Can you work these out from the drawing? Everything is in mm from the part's minimum corner. A direction names the side the tool comes from. Give positions to 0.01 mm unless a question says otherwise; leave off trailing zeros. Order: outer loops, then holes, each group sorted by start corner. A loop starts at its lowest first (then second) coordinate and runs counter-clockwise, first axis right, second up. Notation, with made-up numbers: M -19.75,49.5 L 36.25,49.5 A22 ccw 36.25,81.5 Z; hole C 81,38.25 d8. An arc over 180 degrees is marked long. Answer as a JSON object with one key per item and string values.
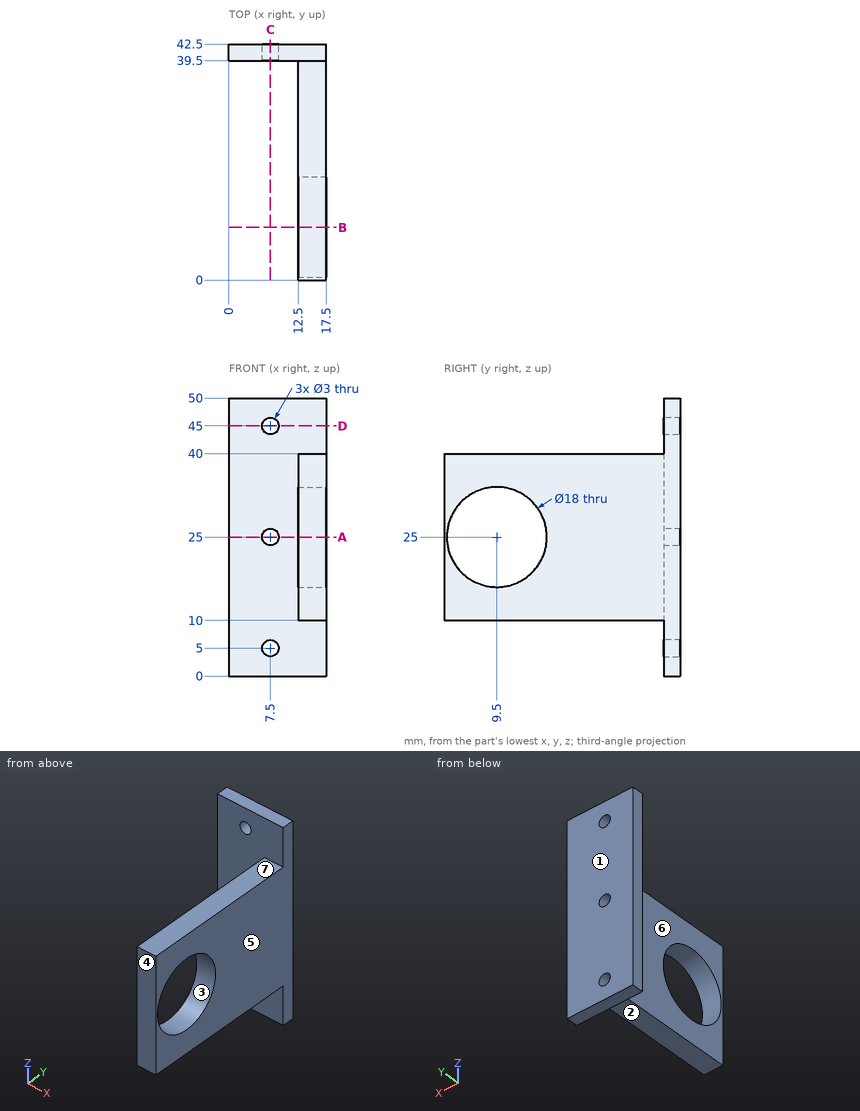
1) I want a section at A-A on z = 25. Write out the boundary of the cut face in (x, y).
Results found:
{"outline": "M 0,39.5 L 6,39.5 L 6,42.5 L 0,42.5 Z; M 9,39.5 L 12.5,39.5 L 12.5,18.5 L 17.5,18.5 L 17.5,42.5 L 9,42.5 Z; M 12.5,0 L 17.5,0 L 17.5,0.5 L 12.5,0.5 Z"}
2) For the marked faces 5, 6 and 7, which set-ups out of +Z, -Z, +X, -X, +Y, -Y let a thin tool reach every point of the face, with its end or its side?
Results found:
{"face 5": "+Z, -Z, +X, +Y, -Y", "face 6": "+Z, -Z, -X, -Y", "face 7": "+Z, +X, -X, -Y"}
3) I want a section at D-D on z = 45. Write out the boundary of the cut face in (x, y).
Results found:
{"outline": "M 0,39.5 L 6,39.5 L 6,42.5 L 0,42.5 Z; M 9,39.5 L 17.5,39.5 L 17.5,42.5 L 9,42.5 Z"}
4) I'm going to push flat-ended pins straight in: pin 1 Ø14.5 at (y, z) = (9.5, 25) entering from +X; pin 2 Ø1.5 at (x, y) = (16, 13) entering from -Z; pin 3 Ø2.5 at (x, y) = (14, 11.5) entering from +Z; pin 4 Ø24 at (y, z) = (10, 21.5) entering from -X. Where does each tip first touch, or does it pass through?
Results found:
{"pin 1": "passes through", "pin 2": "stops at z = 10", "pin 3": "stops at z = 40", "pin 4": "stops at x = 12.5"}
5) Thinking about a two-plate mould opening in Y: for the marked faces 1, 2, 3 and 4, which applies, pulls with the +Y half, pulls with the -Y half, needs draft (parallel to the pull), parting line crosses it, or undercut?
Results found:
{"face 1": "pulls with the +Y half", "face 2": "needs draft", "face 3": "undercut", "face 4": "pulls with the -Y half"}
6) I need wall thicknesses on L1, parallel to X at y = 40.5, z = 45; L2, parallel to Y at x = 11.25, z = 38.5; L3, parallel to Z at x = 16.4, y = 9.5. Which ranges of each line are inside material? Lowest first, please.
Results found:
{"L1": "x = 0 to 6, 9 to 17.5", "L2": "y = 39.5 to 42.5", "L3": "z = 10 to 16, 34 to 40"}
7) I want a section at C-C on x = 7.5. Write out the boundary of the cut face in (y, z), and give its area (3 significant figures).
Results found:
{"outline": "M 39.5,0 L 42.5,0 L 42.5,3.5 L 39.5,3.5 Z; M 39.5,6.5 L 42.5,6.5 L 42.5,23.5 L 39.5,23.5 Z; M 39.5,26.5 L 42.5,26.5 L 42.5,43.5 L 39.5,43.5 Z; M 39.5,46.5 L 42.5,46.5 L 42.5,50 L 39.5,50 Z", "area": "123 mm²"}
8) I want a section at B-B on y = 9.5. Write out the boundary of the cut face in (x, z), and give its area (3 significant figures).
Results found:
{"outline": "M 12.5,10 L 17.5,10 L 17.5,16 L 12.5,16 Z; M 12.5,34 L 17.5,34 L 17.5,40 L 12.5,40 Z", "area": "60.0 mm²"}
